Design review of the part shown in the three views and the two pictorial views. Dimensions are in mm from the part's minimum x, y and z. A direction names the side the tool comes from. Coordinates: 2 decimals unless noted, no trailing zeros. Write each loop counter-clockwise with the first axis right and the second up, starting at its lowest first coordinate (ties: lowest second). Pieces come first, ordered by that corner, then holes. Notation, with made-up numbers: (19, 31.25) - (65, 31.25) arc R12 cw to (65, 43.25) - close; hole circle Ø3 at (75, 34). An arc over 180 degrees is marked (long way). Answer as CSV lines item,"result". Start each with the question number.
Q1. We need section C-C (x = 35.88). Write out the cut boundary in (y, z).
Q2. For line 1 along X through (y, z) = (0.6, 17); line 2 along Y through (x, z) = (12, 10.5); line 3 along X through (y, z) = (10.5, 26), list the stretches that pass through material, from the lowest coordinate up. Write a range as [from, to].
Q3. We need section A-A (y = 15.5). Write out the cut boundary in (x, z).
Q4. We need section B-B (z = 17). Write out the cut boundary in (x, y), plus the area to 3 significant figures.
Q5. We need section D-D (z = 9.5). Write out the cut boundary in (x, y), plus the area to 3 significant figures.
Q6. Clearance check with flat-ended pins moving along their axes: pin 1 (1 mm diameter, centred on y = 9.5, z = 27.5, fed in from -X); pin 2 (8 mm diameter, centred on x = 21.5, y = 12.5, fed in from -Z); pin 3 (3.5 mm diameter, centred on y = 11.5, z = 9.5, fed in from +X). State where each tip first meets the part, or that it passes through.
Q7. Machinability: for the marked faces 1, 2 and 3, which of the approach directions +Z, -Z, +X, -X, +Y, -Y give a long, thin tool a straight path to every point of the face, cutting with its end or side? Answer none if there is none.
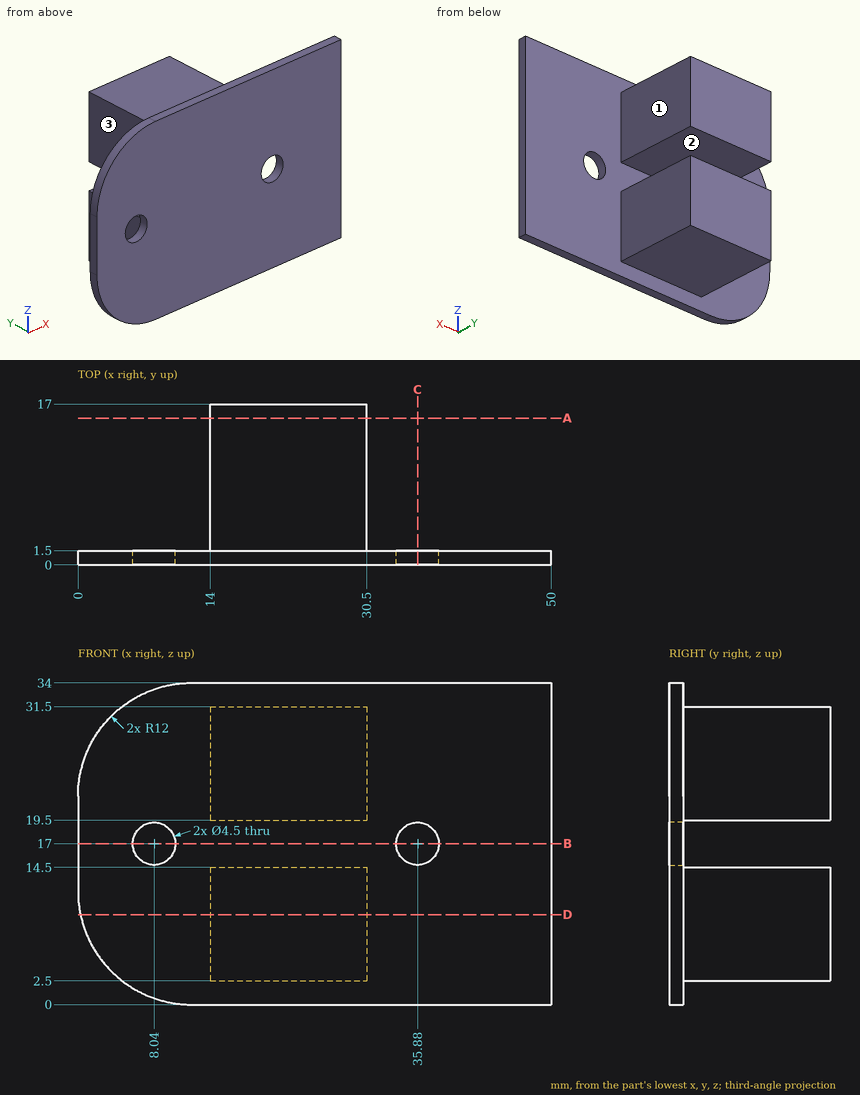
Results list:
1,outline,"(0, 0) - (1.5, 0) - (1.5, 14.75) - (0, 14.75) - close; (0, 19.25) - (1.5, 19.25) - (1.5, 34) - (0, 34) - close"
2,line 1,"x = [0, 5.79], [10.29, 33.63], [38.13, 50]"
2,line 2,"y = [0, 1.5]"
2,line 3,"x = [14, 30.5]"
3,outline,"(14, 2.5) - (30.5, 2.5) - (30.5, 14.5) - (14, 14.5) - close; (14, 19.5) - (30.5, 19.5) - (30.5, 31.5) - (14, 31.5) - close"
4,outline,"(0, 0) - (5.79, 0) - (5.79, 1.5) - (0, 1.5) - close; (10.29, 0) - (33.63, 0) - (33.63, 1.5) - (10.29, 1.5) - close; (38.13, 0) - (50, 0) - (50, 1.5) - (38.13, 1.5) - close"
4,area,"61.5 mm2"
5,outline,"(0.26, 0) - (50, 0) - (50, 1.5) - (30.5, 1.5) - (30.5, 17) - (14, 17) - (14, 1.5) - (0.26, 1.5) - close"
5,area,"330 mm2"
6,pin 1,"stops at x = 14"
6,pin 2,"stops at z = 2.5"
6,pin 3,"stops at x = 30.5"
7,face 1,"+Z, -Z, +X, +Y"
7,face 2,"+X, -X, +Y"
7,face 3,"+Z, -Z, -X, +Y"
